Source: CAD feature listing. Evaluate the final solid. Frame: model axes, mm. A direction names the side the tool comes from. Coordinates: 2 decimals unless noted, no trailing zeros. Write each loop counter-clockwise with the first axis right and the second up, starting at its lowest first coordinate (ties: lowest second). Pieces come first, ordered by that corner, then holes. Notation, with made-up numbers: (56, -29.75) -> (79, -29.75) arc R5 ccw to (79, -22.75) -> close; hole circle Ø6 at (-25.5, 41.25). An arc over 180 degrees is marked (long way). Write item = value, one per line.
from build123d import *

# Parameters (mm, degrees)
F1_DEPTH = 15


with BuildPart() as f1:
    # F0 (on Top) → F1 (new body)
    with BuildSketch(Plane.XY):
        with BuildLine():
            Line((1, 0), (0, 0))
            Line((0, 0), (-19, 0))
            ThreePointArc((-19, 0), (-19.707107, -0.292893), (-20, -1))
            Line((-20, -1), (-20, -2.5))
            ThreePointArc((-20, -2.5), (-19.707107, -3.207107), (-19, -3.5))
            Line((-19, -3.5), (-2, -3.5))
            ThreePointArc((-2, -3.5), (-0.585786, -4.085786), (0, -5.5))
            Line((0, -5.5), (0, -22.8))
            ThreePointArc((0, -22.8), (-0.585786, -24.214214), (-2, -24.8))
            Line((-2, -24.8), (-39, -24.8))
            ThreePointArc((-39, -24.8), (-39.707107, -25.092893), (-40, -25.8))
            Line((-40, -25.8), (-40, -48.8))
            ThreePointArc((-40, -48.8), (-39.707107, -49.507107), (-39, -49.8))
            Line((-39, -49.8), (4, -49.8))
            ThreePointArc((4, -49.8), (4.707107, -49.507107), (5, -48.8))
            Line((5, -48.8), (5, -4))
            ThreePointArc((5, -4), (3.828427, -1.171573), (1, 0))
        make_face()
        with BuildLine():
            ThreePointArc((-36, -31.8), (-35.12132, -29.67868), (-33, -28.8))
            Line((-33, -28.8), (-2, -28.8))
            ThreePointArc((-2, -28.8), (0.12132, -29.67868), (1, -31.8))
            Line((1, -31.8), (1, -42.8))
            ThreePointArc((1, -42.8), (0.12132, -44.92132), (-2, -45.8))
            Line((-2, -45.8), (-33, -45.8))
            ThreePointArc((-33, -45.8), (-35.12132, -44.92132), (-36, -42.8))
            Line((-36, -42.8), (-36, -31.8))
        make_face(mode=Mode.SUBTRACT)
    extrude(amount=F1_DEPTH)


solid = f1.part
1) Cut plane B-B, the plane x = -27.5. Output: boundary loops of the cut face in (y, z), and give its area (3 significant figures).
Answer block:
outline = (-49.8, 0) -> (-45.8, 0) -> (-45.8, 15) -> (-49.8, 15) -> close; (-28.8, 0) -> (-24.8, 0) -> (-24.8, 15) -> (-28.8, 15) -> close
area = 120 mm2
2) Cut plane C-C, the plane z = 10.5. Output: boundary loops of the cut face in (x, y), and give its area (3 significant figures).
Answer block:
outline = (-40, -48.8) arc R1 ccw to (-39, -49.8) -> (4, -49.8) arc R1 ccw to (5, -48.8) -> (5, -4) arc R4 ccw to (1, 0) -> (-19, 0) arc R1 ccw to (-20, -1) -> (-20, -2.5) arc R1 ccw to (-19, -3.5) -> (-2, -3.5) arc R2 cw to (0, -5.5) -> (0, -22.8) arc R2 cw to (-2, -24.8) -> (-39, -24.8) arc R1 ccw to (-40, -25.8) -> close; hole (-36, -42.8) arc R3 ccw to (-33, -45.8) -> (-2, -45.8) arc R3 ccw to (1, -42.8) -> (1, -31.8) arc R3 ccw to (-2, -28.8) -> (-33, -28.8) arc R3 ccw to (-36, -31.8) -> close
area = 695 mm2
3) First-contact query: pin 1 Ø6 at (x, z) = (-32.5, 5) entering from +Y; pin 2 Ø4.5 at (y, z) = (-14.5, 5) entering from -X; pin 3 Ø1.2 at (y, z) = (-1.5, 5.5) entering from -X; pin 4 Ø12 at (x, y) = (-23.5, -15.5) entering from +Z. Flat tips, straight axial feed; report the tip coordinate or a pass-through.
Answer block:
pin_1 = -24.8
pin_2 = 0
pin_3 = -20
pin_4 = through
4) Cut plane A-A, the plane y = -34. Output: boundary loops of the cut face in (x, z).
Answer block:
outline = (-40, 0) -> (-36, 0) -> (-36, 15) -> (-40, 15) -> close; (1, 0) -> (5, 0) -> (5, 15) -> (1, 15) -> close
5) Pull-direction query (Y, two-part tool) for faces 4 (the flat face through (-40, -37, 7)), 5 (the cylindrical face through (-35.14, -29.7, 7.4)), 6 (the flat face through (-9, 0, 7)), 7 (the flat face through (1, -37, 7)); classes: +Y half, -Y half, draft (parallel to the pull), parting line (faces both ways), or undercut.
Answer block:
face_4 = draft
face_5 = undercut
face_6 = +Y half
face_7 = undercut
6) Reachability of faces 1 (the flat face through (-11, -3.5, 7)), 2 (the flat face through (-20, -2, 7)), 3 (the cylindrical face through (0.1, -29.66, 7.4)) from +Z, -Z, +X, -X, +Y, -Y: full face, straight path, thin tool, end or side. Return the list, or none.
Answer block:
face_1 = +Z, -Z, -X
face_2 = +Z, -Z, -X, +Y
face_3 = +Z, -Z
7) Material intervals for probe 1 along Y at (x, z) = (-11, 1.75); probe 2 along Y at (x, z) = (-23.5, 12); probe 3 along X at (y, z) = (-39, 11.5), sorted ascending. Write a range as [from, to].
Answer block:
probe_1 = [-49.8, -45.8], [-28.8, -24.8], [-3.5, 0]
probe_2 = [-49.8, -45.8], [-28.8, -24.8]
probe_3 = [-40, -36], [1, 5]
8) Cut plane D-D, the plane x = -4. Output: boundary loops of the cut face in (y, z).
Answer block:
outline = (-49.8, 0) -> (-45.8, 0) -> (-45.8, 15) -> (-49.8, 15) -> close; (-28.8, 0) -> (-24.8, 0) -> (-24.8, 15) -> (-28.8, 15) -> close; (-3.5, 0) -> (0, 0) -> (0, 15) -> (-3.5, 15) -> close
